Check sheet for the drawn part. Datum: minimum x, y, z corner. Units: mm. A direction names the side the tool comes from. Coordinates: 2 decimals unless noted, no trailing zeros. Write each loop counter-clockwise with the first axis right and the second up, starting at its lowest first coordinate (ties: lowest second). Pieces come first, ordered by that corner, then holes. Notation, with made-up numbers: (27, 53) -> (48, 53) arc R32 cw to (48, 82) -> close; hole circle Ø3 at (36, 80.25). An arc over 180 degrees is marked (long way). Answer in a Markdown table with one row per item.
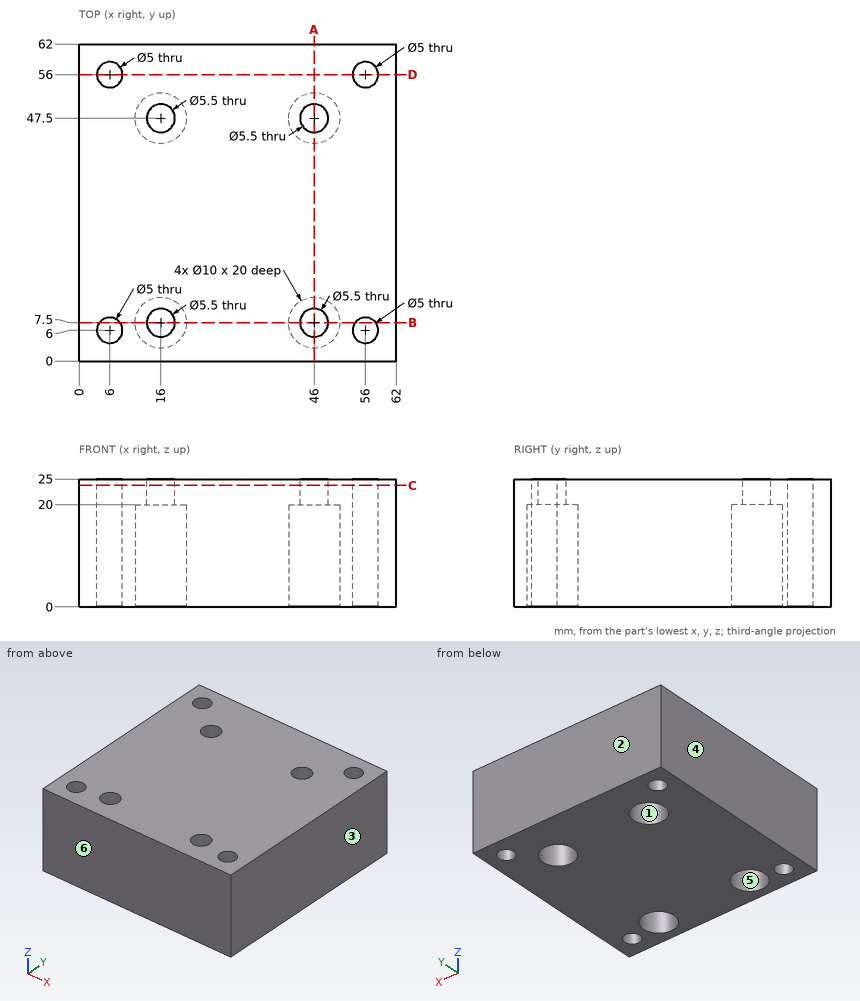
1. Go/stop test with a flat-tipped pin: pin 1 (9 mm diameter, centred on x = 16, y = 47.5, fed in from -Z). Record where the tip stops, or that it passes through.
Findings below:
| item | result |
|---|---|
| pin 1 | stops at z = 20 |
2. Access from +Z, -Z, +X, -X, +Y, -Y to the whole of each face (thin tool, end or side, straight path). Record for the marked faces 1 and 2.
Findings below:
| item | result |
|---|---|
| face 1 | -Z |
| face 2 | +Z, -Z, +X, -X, +Y |
3. Material ranges on probe 1 along Y at (x, z) = (46, 23.6); probe 2 along Y at (x, z) = (56, 18.5); probe 3 along X at (y, z) = (47, 21.5), recorded low to high. Write a range as from..to.
Findings below:
| item | result |
|---|---|
| probe 1 | y = 0..4.75, 10.25..44.75, 50.25..62 |
| probe 2 | y = 0..3.5, 8.5..53.5, 58.5..62 |
| probe 3 | x = 0..13.3, 18.7..43.3, 48.7..62 |
4. Sectioned sample at B-B, the plane y = 7.5. Record the cut outline in (x, z), and give its area (3 significant figures).
Findings below:
| item | result |
|---|---|
| outline | (0, 0) -> (4, 0) -> (4, 25) -> (0, 25) -> close; (8, 0) -> (11, 0) -> (11, 20) -> (13.25, 20) -> (13.25, 25) -> (8, 25) -> close; (18.75, 20) -> (21, 20) -> (21, 0) -> (41, 0) -> (41, 20) -> (43.25, 20) -> (43.25, 25) -> (18.75, 25) -> close; (48.75, 20) -> (51, 20) -> (51, 0) -> (54, 0) -> (54, 25) -> (48.75, 25) -> close; (58, 0) -> (62, 0) -> (62, 25) -> (58, 25) -> close |
| area | 895 mm² |
5. Release check for a two-part mould opening along X. For the marked faces 3, 4, 5 and 6 record: released by +X, released by -X, zero draft, split by the parting line, or undercut.
Findings below:
| item | result |
|---|---|
| face 3 | released by +X |
| face 4 | released by -X |
| face 5 | undercut |
| face 6 | zero draft |
6. Sectioned sample at C-C, the plane z = 23.75. Count the separate pieces of the cut face and the enclosed holes in it, and give its area (3 significant figures).
Findings below:
| item | result |
|---|---|
| separate pieces | 1 |
| enclosed holes | 8 |
| area | 3,670 mm² |
7. Sectioned sample at A-A, the plane x = 46. Record the cut outline in (y, z), and give its area (4 significant figures).
Findings below:
| item | result |
|---|---|
| outline | (0, 0) -> (2.5, 0) -> (2.5, 20) -> (4.75, 20) -> (4.75, 25) -> (0, 25) -> close; (10.25, 20) -> (12.5, 20) -> (12.5, 0) -> (42.5, 0) -> (42.5, 20) -> (44.75, 20) -> (44.75, 25) -> (10.25, 25) -> close; (50.25, 20) -> (52.5, 20) -> (52.5, 0) -> (62, 0) -> (62, 25) -> (50.25, 25) -> close |
| area | 1,095 mm² |
8. Sectioned sample at D-D, the plane y = 56. Record the cut outline in (x, z).
Findings below:
| item | result |
|---|---|
| outline | (0, 0) -> (3.5, 0) -> (3.5, 25) -> (0, 25) -> close; (8.5, 0) -> (53.5, 0) -> (53.5, 25) -> (8.5, 25) -> close; (58.5, 0) -> (62, 0) -> (62, 25) -> (58.5, 25) -> close |
